from build123d import *

# Parameters (mm, degrees)
F0_W         = 19.05
F0_H         = 19.05
F1_DEPTH     = 19.05
F2_R         = 2.54
F3_T1_DEPTH  = 28.575
F3_T4_ANGLE  = 90
F3_T6_ANGLE  = 90
F3_T8_ANGLE  = 90
F3_T10_ANGLE = 90
F4_R         = 2.54
F5_DEPTH     = 6.35


# Not quite as in the source:
# - a fillet or chamfer that OpenCascade refuses, or shapes differently, is made with other operations: its cross-section is extruded or revolved along the edge and cut away or added


with BuildPart() as f1:
    # F0 (on Top) → F1 (new body)
    with BuildSketch(Plane.XY):
        with Locations((-40.0474531332, 35.1082887501)):
            Rectangle(F0_W, F0_H)
    extrude(amount=F1_DEPTH)

    # F2
    f2_edges = [f1.edges().sort_by_distance(p)[0] for p in [
        (-40.047453, 44.633289, 19.05),
        (-49.572453, 35.108289, 19.05),
        (-40.047453, 25.583289, 19.05),
        (-30.522453, 35.108289, 19.05),
    ]]
    fillet(f2_edges, radius=F2_R)

    # F3: fillet of radius 3.81 on 4 edges, made by hand

    # F3_s2 → F3_t1 (cut)
    with BuildSketch(Plane.XY.offset(-9.525)):
        with BuildLine():
            ThreePointArc((-49.5724531332, 29.3932887501), (-48.4565299695, 26.6992119137), (-45.7624531332, 25.5832887501))
            Line((-45.7624531332, 25.5832887501), (-49.5724531332, 25.5832887501))
            Line((-49.5724531332, 25.5832887501), (-49.5724531332, 29.3932887501))
        make_face()
        with BuildLine():
            ThreePointArc((-45.7624531332, 44.6332887501), (-48.4565299695, 43.5173655864), (-49.5724531332, 40.8232887501))
            Line((-49.5724531332, 40.8232887501), (-49.5724531332, 44.6332887501))
            Line((-49.5724531332, 44.6332887501), (-45.7624531332, 44.6332887501))
        make_face()
        with BuildLine():
            ThreePointArc((-30.5224531332, 29.3932887501), (-31.6383762969, 26.6992119137), (-34.3324531332, 25.5832887501))
            Line((-34.3324531332, 25.5832887501), (-30.5224531332, 25.5832887501))
            Line((-30.5224531332, 25.5832887501), (-30.5224531332, 29.3932887501))
        make_face()
        with BuildLine():
            ThreePointArc((-34.3324531332, 44.6332887501), (-31.6383762969, 43.5173655864), (-30.5224531332, 40.8232887501))
            Line((-30.5224531332, 40.8232887501), (-30.5224531332, 44.6332887501))
            Line((-30.5224531332, 44.6332887501), (-34.3324531332, 44.6332887501))
        make_face()
    extrude(amount=F3_T1_DEPTH, mode=Mode.SUBTRACT)

    # F3_s3 → F3_t4 (revolve, cut)
    with BuildSketch(Plane.XZ.offset(-40.8232887501)):
        with BuildLine():
            ThreePointArc((-33.0624531332, 19.05), (-31.266401909, 18.3060512242), (-30.5224531332, 16.51))
            Line((-30.5224531332, 16.51), (-30.5224531332, 19.05))
            Line((-30.5224531332, 19.05), (-33.0624531332, 19.05))
        make_face()
    revolve(axis=Axis((-34.3324531332, 40.8232887501, 19.05), (0, 0, 1)), revolution_arc=F3_T4_ANGLE, mode=Mode.SUBTRACT)

    # F3_s5 → F3_t6 (revolve, cut)
    with BuildSketch(Plane.YZ.offset(-34.3324531332)):
        with BuildLine():
            ThreePointArc((28.1232887501, 19.05), (26.3272375258, 18.3060512242), (25.5832887501, 16.51))
            Line((25.5832887501, 16.51), (25.5832887501, 19.05))
            Line((25.5832887501, 19.05), (28.1232887501, 19.05))
        make_face()
    revolve(axis=Axis((-34.3324531332, 29.3932887501, 19.05), (0, 0, 1)), revolution_arc=F3_T6_ANGLE, mode=Mode.SUBTRACT)

    # F3_s7 → F3_t8 (revolve, cut)
    with BuildSketch(Plane.YZ.offset(-45.7624531332)):
        with BuildLine():
            ThreePointArc((42.0932887501, 19.05), (43.8893399743, 18.3060512242), (44.6332887501, 16.51))
            Line((44.6332887501, 16.51), (44.6332887501, 19.05))
            Line((44.6332887501, 19.05), (42.0932887501, 19.05))
        make_face()
    revolve(axis=Axis((-45.7624531332, 40.8232887501, 19.05), (0, 0, 1)), revolution_arc=F3_T8_ANGLE, mode=Mode.SUBTRACT)

    # F3_s9 → F3_t10 (revolve, cut)
    with BuildSketch(Plane.XZ.offset(-29.3932887501)):
        with BuildLine():
            ThreePointArc((-47.0324531332, 19.05), (-48.8285043574, 18.3060512242), (-49.5724531332, 16.51))
            Line((-49.5724531332, 16.51), (-49.5724531332, 19.05))
            Line((-49.5724531332, 19.05), (-47.0324531332, 19.05))
        make_face()
    revolve(axis=Axis((-45.7624531332, 29.3932887501, 19.05), (0, 0, 1)), revolution_arc=F3_T10_ANGLE, mode=Mode.SUBTRACT)

    # F4 (on face) → F5 (join)
    with BuildSketch(Plane(origin=(0, 0, 0), x_dir=(1, 0, 0), z_dir=(0, 0, -1))):
        with Locations((-40.0474531332, -35.1082887501)):
            Circle(F4_R)
    extrude(amount=F5_DEPTH)


solid = f1.part
Can you work these out from the model? Positions are in its coordinate system, mm. A direction names the side the tool comes from. Round coordinates to 2 decimals unless told otherwise and drop trailing zeros. Order: outer loops, then holes, each group sorted by start corner. A loop starts at its lowest first (then second) coordinate and runs counter-clockwise, first axis right, second up. Notation, with made-up numbers: M -38,-6.5 L -34,-6.5 A31 cw -34,20.5 Z; hole C -24,13 d9. An arc over 180 degrees is marked long. Use a Markdown table: item, result.
1) If I drill on line 1 along Z through (x, y) = (-39.25, 38.5); line 2 along X through (y, z) = (36, -3.25), over which ranges is the centre line in solid material (lowest first)?
Geometry says:
| item | result |
|---|---|
| line 1 | z = 0 to 19.05 |
| line 2 | x = -42.43 to -37.67 |
2) I'm going to push a flat-ended pin straight in: P1, Ø1, axis at y = 28, z = 11, coming from the +X side. Where does the tip first touch, or does it pass through?
Geometry says:
| item | result |
|---|---|
| P1 | stops at x = -30.63 |
3) Imagine slicing it at B-B (x = -35.25). List the corners of the cut face in (y, z) for me.
Geometry says:
| item | result |
|---|---|
| outline | M 25.58,0 L 44.63,0 L 44.63,16.51 A2.54 ccw 42.09,19.05 L 28.12,19.05 A2.54 ccw 25.58,16.51 Z |
4) Imagine slicing it at A-A (z = 5.25). List the corners of the cut face in (x, y) for me.
Geometry says:
| item | result |
|---|---|
| outline | M -49.57,29.39 A3.81 ccw -45.76,25.58 L -34.33,25.58 A3.81 ccw -30.52,29.39 L -30.52,40.82 A3.81 ccw -34.33,44.63 L -45.76,44.63 A3.81 ccw -49.57,40.82 Z |
5) On a 3-axis mill with a long thin cutter (end or side, diameter ignored), from which of +Z, -Z, +X, -X, +Y, -Y can I reach the whole of each face in a straight line? I mean faces 1 (the face through (-48.427, 43.547, 8.139)), 2 (the face through (-40.38, 32.59, -3.13)). Say none if no direction works.
Geometry says:
| item | result |
|---|---|
| face 1 | +Z, -Z, -X, +Y |
| face 2 | -Z |
6) Imagine slicing it at D-D (y = 35.5). List the corners of the cut face in (x, z) for me, then the cut area to 3 significant figures.
Geometry says:
| item | result |
|---|---|
| outline | M -49.57,0 L -42.56,0 L -42.56,-6.35 L -37.54,-6.35 L -37.54,0 L -30.52,0 L -30.52,16.51 A2.54 ccw -33.06,19.05 L -47.03,19.05 A2.54 ccw -49.57,16.51 Z |
| area | 392 mm² |
7) Imagine slicing it at C-C (y = 39.5). List the corners of the cut face in (x, z) for me, then the cut area to 3 significant figures.
Geometry says:
| item | result |
|---|---|
| outline | M -49.57,0 L -30.52,0 L -30.52,16.51 A2.54 ccw -33.06,19.05 L -47.03,19.05 A2.54 ccw -49.57,16.51 Z |
| area | 360 mm² |
